```python
from build123d import *

# Parameters (mm, degrees)
F0_R     = 17.85
F1_DEPTH = 1.2
F2_R     = 12.75
F3_DEPTH = 6
F4_W     = 9.2
F4_H     = 18.8
F5_DEPTH = 7.201
F7_DEPTH = 6.7
F9_DEPTH = 4


with BuildPart() as f1:
    # F0 (on Top) → F1 (new body)
    with BuildSketch(Plane.XY):
        Circle(F0_R)
    extrude(amount=F1_DEPTH)

    # F2 (on face) → F3 (join)
    with BuildSketch(Plane.XY.offset(1.2)):
        Circle(F2_R)
    extrude(amount=F3_DEPTH)

    # F4 (on face) → F5 (cut, through all)
    with BuildSketch(Plane.XY.offset(7.2)):
        Rectangle(F4_W, F4_H)
    extrude(amount=-F5_DEPTH, mode=Mode.SUBTRACT)

    # F6 (on face) → F7 (cut)
    with BuildSketch(Plane.XY.offset(7.2)):
        with BuildLine():
            Line((5.4, 10.35), (-5.4, 10.35))
            Line((-5.4, 10.35), (-5.4, 7.4))
            ThreePointArc((-5.4, 7.4), (-5, 7), (-5.4, 6.6))
            Line((-5.4, 6.6), (-5.4, -6.6))
            ThreePointArc((-5.4, -6.6), (-5, -7), (-5.4, -7.4))
            Line((-5.4, -7.4), (-5.4, -10.35))
            Line((-5.4, -10.35), (5.4, -10.35))
            Line((5.4, -10.35), (5.4, -7.4))
            ThreePointArc((5.4, -7.4), (5, -7), (5.4, -6.6))
            Line((5.4, -6.6), (5.4, 6.6))
            ThreePointArc((5.4, 6.6), (5, 7), (5.4, 7.4))
            Line((5.4, 7.4), (5.4, 10.35))
        make_face()
    extrude(amount=-F7_DEPTH, mode=Mode.SUBTRACT)

    # F8 (on face) → F9 (cut)
    with BuildSketch(Plane.XY.offset(7.2)):
        with BuildLine():
            Line((4.4, 10.85), (-4.4, 10.85))
            ThreePointArc((-4.4, 10.85), (-5.46066, 10.41066), (-5.9, 9.35))
            Line((-5.9, 9.35), (-5.9, -9.35))
            ThreePointArc((-5.9, -9.35), (-5.46066, -10.41066), (-4.4, -10.85))
            Line((-4.4, -10.85), (4.4, -10.85))
            ThreePointArc((4.4, -10.85), (5.46066, -10.41066), (5.9, -9.35))
            Line((5.9, -9.35), (5.9, 9.35))
            ThreePointArc((5.9, 9.35), (5.46066, 10.41066), (4.4, 10.85))
        make_face()
    extrude(amount=-F9_DEPTH, mode=Mode.SUBTRACT)


solid = f1.part
```
Verification items for the finished model (mm, model axes). Coordinates: 2 decimals unless noted, no trailing zeros. Loops run counter-clockwise (first coordinate to the right, second up) from the corner with the lowest first, then second, coordinate; pieces in that order, holes last. Notation, with made-up numbers: (-19.75, 45) -> (-2.75, 45) arc R9 cw to (-2.75, 56) -> close; hole circle Ø7 at (19.5, 59.25). An arc over 180 degrees is marked (long way). Answer in a Markdown table with one row per item. Add a question column.
1. Section check D-D, the plane x = 11. Enter the section's corners in (y, z).
2. Depth check by flat-ended pin: P1, Ø0.6, axis at y = 4, z = 0.5, coming from the +X side; P2, Ø0.8, axis at x = -2.5, z = 2, coming from the +Y side; P3, Ø1, axis at x = 6.5, z = 2.5, coming from the -Y side. Enter the tip coordinate at first touch or a pass-through.
3. Draft check along X on faces 1 (the face through (8, 0, 7.2)), 2 (the face through (0, -10.85, 5)), 3 (the face through (-2.764, -12.447, 4.158)). Enter one of: +X half, -X half, draft (parallel to the pull), parting line (faces both ways), or undercut.
4. Section check B-B, the plane x = 2. Enter the section's corners in (y, z), then the cut area to 3 significant figures.
5. Material ranges on probe 1 along Z at (x, y) = (12, 7); probe 2 along Z at (x, y) = (-5.5, -3); probe 3 along X at (y, z) = (-10.5, 6), recorded low to high. Write a range as [from, to].
6. Section check A-A, the plane y = 0. Enter the section's corners in (x, z).
7. Section check C-C, the plane z = 6.5. Enter the section's corners in (x, y), then the cut area to 3 significant figures.
Derived:
| question | item | result |
|---|---|---|
| 1 | outline | (-14.06, 0) -> (14.06, 0) -> (14.06, 1.2) -> (6.45, 1.2) -> (6.45, 7.2) -> (-6.45, 7.2) -> (-6.45, 1.2) -> (-14.06, 1.2) -> close |
| 2 | P1 | stops at x = 17.46 |
| 2 | P2 | stops at y = 12.58 |
| 2 | P3 | stops at y = -11.25 |
| 3 | face 1 | draft |
| 3 | face 2 | undercut |
| 3 | face 3 | parting line |
| 4 | outline | (-17.74, 0) -> (-9.4, 0) -> (-9.4, 0.5) -> (-10.35, 0.5) -> (-10.35, 3.2) -> (-10.85, 3.2) -> (-10.85, 7.2) -> (-12.59, 7.2) -> (-12.59, 1.2) -> (-17.74, 1.2) -> close; (9.4, 0) -> (17.74, 0) -> (17.74, 1.2) -> (12.59, 1.2) -> (12.59, 7.2) -> (10.85, 7.2) -> (10.85, 3.2) -> (10.35, 3.2) -> (10.35, 0.5) -> (9.4, 0.5) -> close |
| 4 | area | 41.6 mm² |
| 5 | probe 1 | z = [0, 1.2] |
| 5 | probe 2 | z = [0, 3.2] |
| 5 | probe 3 | x = [-7.23, -5.36], [5.36, 7.23] |
| 6 | outline | (-17.85, 0) -> (-4.6, 0) -> (-4.6, 0.5) -> (-5.4, 0.5) -> (-5.4, 3.2) -> (-5.9, 3.2) -> (-5.9, 7.2) -> (-12.75, 7.2) -> (-12.75, 1.2) -> (-17.85, 1.2) -> close; (4.6, 0) -> (17.85, 0) -> (17.85, 1.2) -> (12.75, 1.2) -> (12.75, 7.2) -> (5.9, 7.2) -> (5.9, 3.2) -> (5.4, 3.2) -> (5.4, 0.5) -> (4.6, 0.5) -> close |
| 7 | outline | circle Ø25.5 at (0, 0); hole (-5.9, -9.35) arc R1.5 ccw to (-4.4, -10.85) -> (4.4, -10.85) arc R1.5 ccw to (5.9, -9.35) -> (5.9, 9.35) arc R1.5 ccw to (4.4, 10.85) -> (-4.4, 10.85) arc R1.5 ccw to (-5.9, 9.35) -> close |
| 7 | area | 257 mm² |
